Autodesk Inventor part; units mm, degrees
sketch "Эскиз1" plane through (0, 0, 0) normal (0, 1, 0) x (-1, 0, 0)
  line L0 (230, -325) -> (-230, -325)
  line L1 (-230, -325) -> (-230, 325)
  line L2 (-230, 325) -> (230, 325)
  line L3 (230, 325) -> (230, -325)
  line L4 (230, -325) -> (-230, 325) construction
  line L5 (-230, -325) -> (230, 325) construction
  line L6 (-230, -325) -> (-170, -325)
  line L7 (-170, -325) -> (-170, -295)
  line L8 (-170, -295) -> (-230, -295)
  line L9 (-230, -295) -> (-230, -325)
  line L10 (-230, -325) -> (-200, -325)
  line L11 (-200, -325) -> (-200, -265)
  line L12 (-200, -265) -> (-230, -265)
  line L13 (-230, -265) -> (-230, -325)
  line L14 (-230, 0) -> (230, 0) construction
  line L15 (0, -325) -> (0, 325) construction
  line L16 (-230, 325) -> (-170, 325)
  line L17 (-170, 325) -> (-170, 295)
  line L18 (-170, 295) -> (-230, 295)
  line L19 (-230, 295) -> (-230, 325)
  line L20 (-230, 325) -> (-200, 325)
  line L21 (-200, 325) -> (-200, 265)
  line L22 (-200, 265) -> (-230, 265)
  line L23 (-230, 265) -> (-230, 325)
  line L24 (230, -325) -> (170, -325)
  line L25 (170, -325) -> (170, -295)
  line L26 (170, -295) -> (230, -295)
  line L27 (230, -295) -> (230, -325)
  line L28 (230, -325) -> (200, -325)
  line L29 (200, -325) -> (200, -265)
  line L30 (200, -265) -> (230, -265)
  line L31 (230, -265) -> (230, -325)
  line L32 (170, 295) -> (230, 295)
  line L33 (230, 325) -> (170, 325)
  line L34 (170, 325) -> (170, 295)
  line L35 (230, 295) -> (230, 325)
  line L36 (230, 325) -> (200, 325)
  line L37 (200, 325) -> (200, 265)
  line L38 (230, 265) -> (230, 325)
  line L39 (200, 265) -> (230, 265)
  point P0 (0, 0)
  point P1 (200, 295)
  point P2 (-200, 295)
  point P3 (-200, -295)
  point P4 (200, -295)
  dimension "d0" = 650
  dimension "d1" = 460
  dimension "d2" = 30
  dimension "d3" = 60
extrude "Выдавливание1" add sketch "Эскиз1" along normal blind 3 contours L0 L7 L8 L11 L12 L1 L22 L21 L18 L17 L2 L34 L32 L37 L39 L3 L30 L29 L26 L25
properties part number "Фанера платформы"
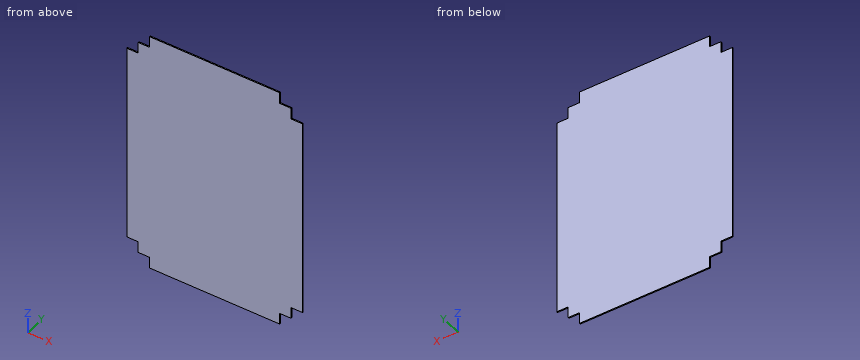
The model under review builds one solid part; all positions refer to its coordinate system, in mm. Round coordinates to 2 decimals unless told otherwise and drop trailing zeros. Order: outer loops, then holes, each group sorted by start corner. A loop starts at its lowest first (then second) coordinate and runs counter-clockwise, first axis right, second up. Notation, with made-up numbers: M -37.5,62 L 3.5,62 A25 ccw 3.5,82 Z; hole C 84,44 d4. An arc over 180 degrees is marked long. Use a Markdown table: item, result.
1) Wall thickness on line 1 along Z through (x, y) = (-198, 2.25); line 2 along X through (y, z) = (1.55, -273): over which ranges is each line inside the solid? List them lowest first. Write a range as [from, to].
Report:
| item | result |
|---|---|
| line 1 | [-295, 295] |
| line 2 | [-200, 200] |
2) Consider section B-B (z = 284.5). Write out the cut boundary in (x, y), then the cut area to 3 significant figures.
Report:
| item | result |
|---|---|
| outline | M -200,0 L 200,0 L 200,3 L -200,3 Z |
| area | 1,200 mm^2 |
3) Insertion check: pin 1 (0.9 mm diameter, centred on y = 2, z = 309.5, fed in from -X); pin 2 (1.5 mm diameter, centred on x = 210.5, y = 1, fed in from +Z); pin 3 (1.5 mm diameter, centred on y = 2, z = -286, fed in from +X). Each pin has a flat end and moves straight along its axis. Give the tip position at first contact, or say it passes through.
Report:
| item | result |
|---|---|
| pin 1 | x = -170 |
| pin 2 | z = 265 |
| pin 3 | x = 200 |
4) Consider section A-A (y = 1.75). Write out the cut boundary in (x, z).
Report:
| item | result |
|---|---|
| outline | M -230,-265 L -200,-265 L -200,-295 L -170,-295 L -170,-325 L 170,-325 L 170,-295 L 200,-295 L 200,-265 L 230,-265 L 230,265 L 200,265 L 200,295 L 170,295 L 170,325 L -170,325 L -170,295 L -200,295 L -200,265 L -230,265 Z |
5) Consider section C-C (x = -180.5). Write out the cut boundary in (y, z).
Report:
| item | result |
|---|---|
| outline | M 0,-295 L 3,-295 L 3,295 L 0,295 Z |
